Check sheet for the drawn part. Datum: minimum x, y, z corner. Units: mm. A direction names the side the tool comes from. Coordinates: 2 decimals unless noted, no trailing zeros. Write each loop counter-clockwise with the first axis right and the second up, starting at its lowest first coordinate (ties: lowest second). Pieces come first, ordered by that corner, then holes. Notation, with made-up numbers: (66, 49.5) - (124, 49.5) arc R16 ccw to (124, 60.5) - close; hole circle Ø8 at (-35, -37). An arc over 180 degrees is marked (long way). Answer as CSV lines item,"result". Start each with the question number.
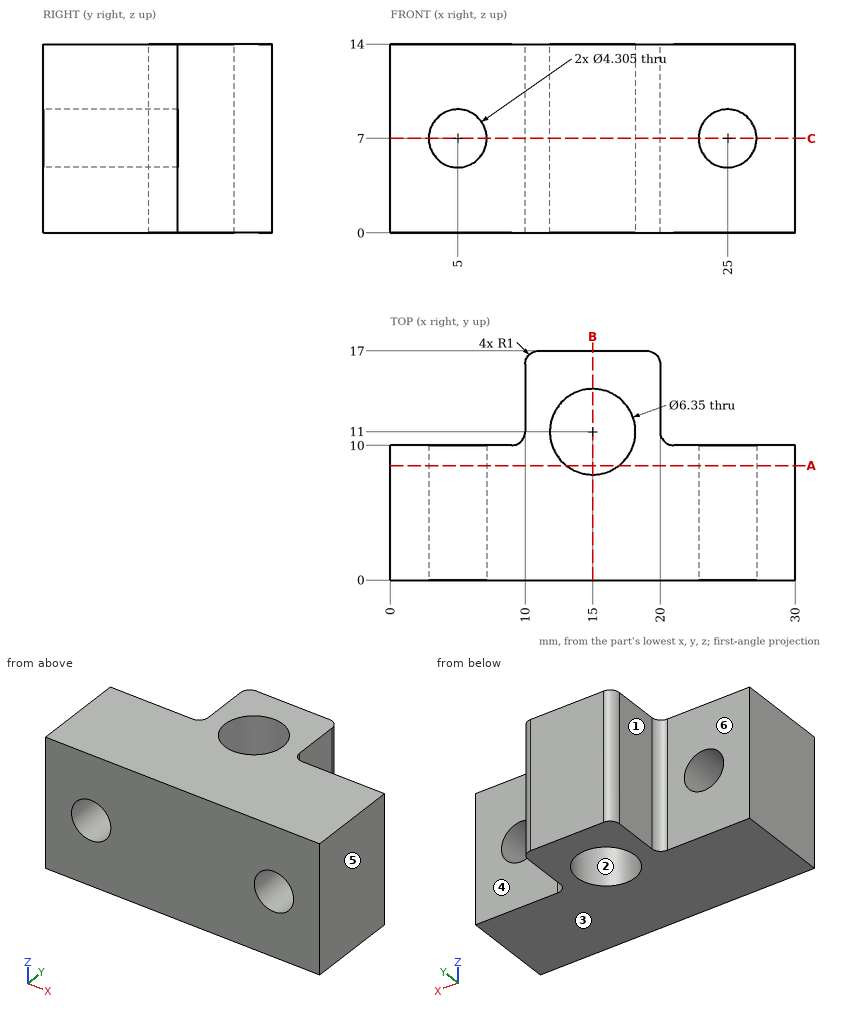
(1) Cross-section at B-B on x = 15. Record the boundary of the cut face in (y, z) (1 decimal).
(2) Go/stop test with flat-tipped pins: P1, Ø4, axis at y = 12.5, z = 6.5, coming from the -X side; P2, Ø8, axis at x = 13.5, y = 2, coming from the -Z side; P3, Ø8, axis at x = 3, z = 9, coming from the +Y side; P4, Ø2, axis at x = 13.5, y = 12, coming from the -Z side. Record where each tip stops, or that it passes through.
(3) Tool access check on the marked faces 4, 5 and 6. Record the directions out of +Z, -Z, +X, -X, +Y, -Y that give a thin tool (end or side, any length) a straight path to the whole face; none if there is none.
(4) Cross-section at A-A on y = 8.5. Record the boundary of the cut face in (x, z) (1 decimal).
(5) Material ranges on probe 1 along Z at (x, y) = (25, 6.5); probe 2 along Y at (x, z) = (15, 7.75) (1 decimal); probe 3 along Y at (x, z) = (3.5, 12.5), recorded low to high. Write a range as from..to.
(6) Release check for a two-part mould opening along X. For the marked faces 1, 2 and 3 record: pulls with the +X half, pulls with the -X half, needs draft (parallel to the pull), parting line crosses it, or undercut.
(7) Cross-section at C-C on z = 7. State how many separate pieces and enclosed holes the cut face has, plus the area to 3 significant figures.
Checked values:
1,outline,"(0, 0) - (7.8, 0) - (7.8, 14) - (0, 14) - close; (14.2, 0) - (17, 0) - (17, 14) - (14.2, 14) - close"
2,P1,"x = 9.87"
2,P2,"z = 0"
2,P3,"y = 10"
2,P4,"through"
3,face 4,"+Z, -Z, +X, +Y"
3,face 5,"+Z, -Z, +X, +Y, -Y"
3,face 6,"+Z, -Z, -X, +Y"
4,outline,"(0, 0) - (13, 0) - (13, 14) - (0, 14) - close; (17, 0) - (30, 0) - (30, 14) - (17, 14) - close; hole circle Ø4.3 at (5, 7); hole circle Ø4.3 at (25, 7)"
5,probe 1,"0..4.85, 9.15..14"
5,probe 2,"0..7.8, 14.2..17"
5,probe 3,"0..10"
6,face 1,"pulls with the -X half"
6,face 2,"undercut"
6,face 3,"needs draft"
7,separate pieces,"3"
7,enclosed holes,"1"
7,area,"252 mm^2"
